Verification items for this drawing (mm, ordinates from the low corner). Coordinates: 2 decimals unless noted, no trailing zeros. Write each question's results on one line, items separated by ' | '.
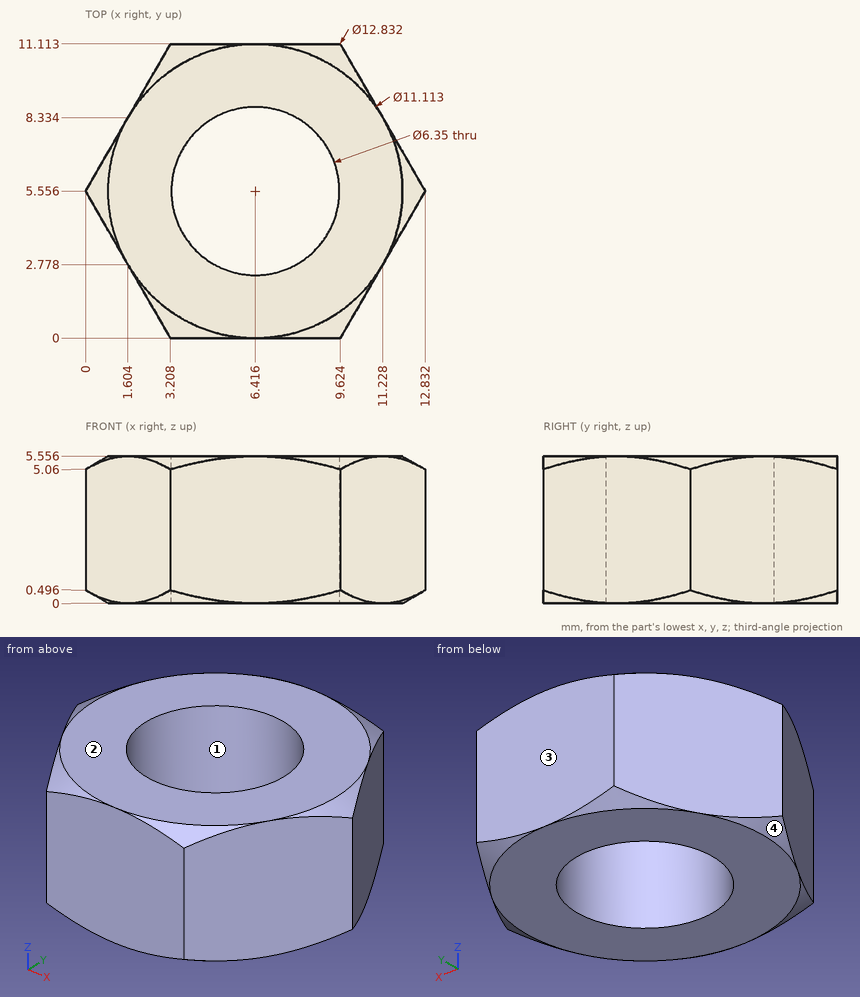
Q1. Mould release check, pull along Y, two halves, no side actions. Record for the marked faces 1, 2, 3 and 4: pulls with the +Y half, pulls with the -Y half, needs draft (parallel to the pull), parting line crosses it, or undercut.
Geometry check:
face 1: undercut | face 2: needs draft | face 3: pulls with the +Y half | face 4: parting line crosses it
Q2. Scan lines: probe 1 along X at (y, z) = (5.25, 1.8) (1 decimal); probe 2 along X at (y, z) = (8.25, 2.65) (1 decimal); probe 3 along Y at (x, z) = (6.5, 0.5). Record each from-to range of solid material in increasing order.
Geometry check:
probe 1: x = 0.2 to 3.3, 9.6 to 12.7 | probe 2: x = 1.6 to 4.7, 8.1 to 11.3 | probe 3: y = 0 to 2.38, 8.73 to 11.11
Q3. Depth check by flat-ended pin: P1, Ø1.5, axis at y = 3.5, z = 5, coming from the +X side; P2, Ø4, axis at x = 6.42, y = 5.56, coming from the -Z side (1 decimal); P3, Ø1.5, axis at y = 10, z = 3, coming from the +X side; P4, Ø4, axis at x = 9.5, y = 5.5, coming from the +Z side. Enter the tip coordinate at first touch or a pass-through.
Geometry check:
P1: stops at x = 12.08 | P2: passes through | P3: stops at x = 10.7 | P4: stops at z = 5.56
